CAD build for the part. Positions are in the model's coordinates, mm. Face numbers are marked on the shaded views. Round coordinates to 2 decimals unless told otherwise and drop trailing zeros. Loops run counter-clockwise (first coordinate to the right, second up) from the corner with the lowest first, then second, coordinate; pieces in that order, holes last. Notation, with made-up numbers: M 55.5,67 L 103.5,67 A21 ccw 103.5,98 Z; hole C -14,-25.5 d5. An arc over 180 degrees is marked long. Use a Markdown table: item, result. Add a question column.
(1) Flat gauge pin, fed straight in: P1, Ø4.5, axis at x = 0, y = -12.7, coming from the +Z side. Where does the tip first touch, or does it go through?
(2) Band-saw the part on B-B, the plane y = 12.7. Write the cut outline in (x, z), and give its area (3 significant figures).
(3) Band-saw the part on C-C, the plane z = 2.75. Write the cut outline in (x, y).
(4) Two-plate mould, pull along X, no slides. Class the marked faces 1, 2, 3 and 4: released by +X, released by -X, zero draft, split by the parting line, or undercut.
(5) Band-saw the part on A-A, the plane x = 0. Write the cut outline in (y, z).
(6) Wall check: L1, parallel to Y at x = 0, z = 5; L2, parallel to X at y = -12.7, z = 4.5; L3, parallel to X at y = -11, z = 6.25. Give the ranges that are in metal, low to high.
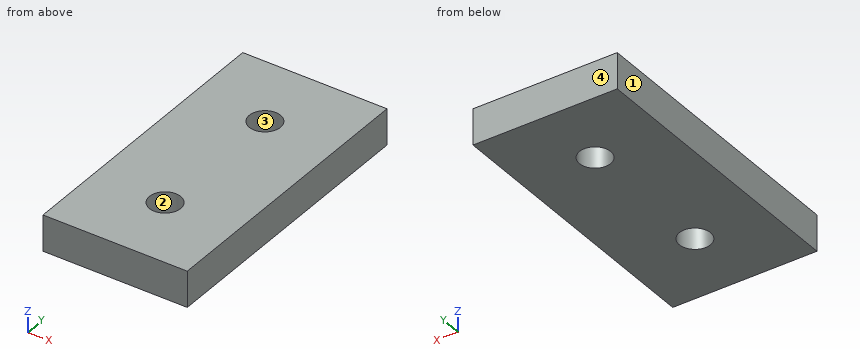
from build123d import *

# Parameters (mm, degrees)
ESQUISSE1_W             = 25.4
ESQUISSE1_H             = 50.8
BOSS_EXTRU_1_DEPTH      = 6.35
ESQUISSE2_R             = 2.75
ENL_V_MAT_EXTRU_1_DEPTH = 6.35


with BuildPart() as part:
    # Esquisse1 → Boss.-Extru.1 (new body)
    with BuildSketch(Plane.XY):
        Rectangle(ESQUISSE1_W, ESQUISSE1_H)
    extrude(amount=BOSS_EXTRU_1_DEPTH)

    # Esquisse2 → Enlèv. mat.-Extru.1 (cut)
    with BuildSketch(Plane.XY.offset(6.35)):
        with Locations((0, 12.7)):
            Circle(ESQUISSE2_R)
        with Locations(Location((0, -12.7, 0), (0, 0, 180))):
            Circle(ESQUISSE2_R)
    extrude(amount=-ENL_V_MAT_EXTRU_1_DEPTH, mode=Mode.SUBTRACT)


solid = part.part
Return value:
| question | item | result |
|---|---|---|
| 1 | P1 | through |
| 2 | outline | M -12.7,0 L -2.75,0 L -2.75,6.35 L -12.7,6.35 Z; M 2.75,0 L 12.7,0 L 12.7,6.35 L 2.75,6.35 Z |
| 2 | area | 126 mm^2 |
| 3 | outline | M -12.7,-25.4 L 12.7,-25.4 L 12.7,25.4 L -12.7,25.4 Z; hole C 0,-12.7 d5.5; hole C 0,12.7 d5.5 |
| 4 | face 1 | released by -X |
| 4 | face 2 | undercut |
| 4 | face 3 | undercut |
| 4 | face 4 | zero draft |
| 5 | outline | M -25.4,0 L -15.45,0 L -15.45,6.35 L -25.4,6.35 Z; M -9.95,0 L 9.95,0 L 9.95,6.35 L -9.95,6.35 Z; M 15.45,0 L 25.4,0 L 25.4,6.35 L 15.45,6.35 Z |
| 6 | L1 | -25.4 to -15.45, -9.95 to 9.95, 15.45 to 25.4 |
| 6 | L2 | -12.7 to -2.75, 2.75 to 12.7 |
| 6 | L3 | -12.7 to -2.16, 2.16 to 12.7 |
